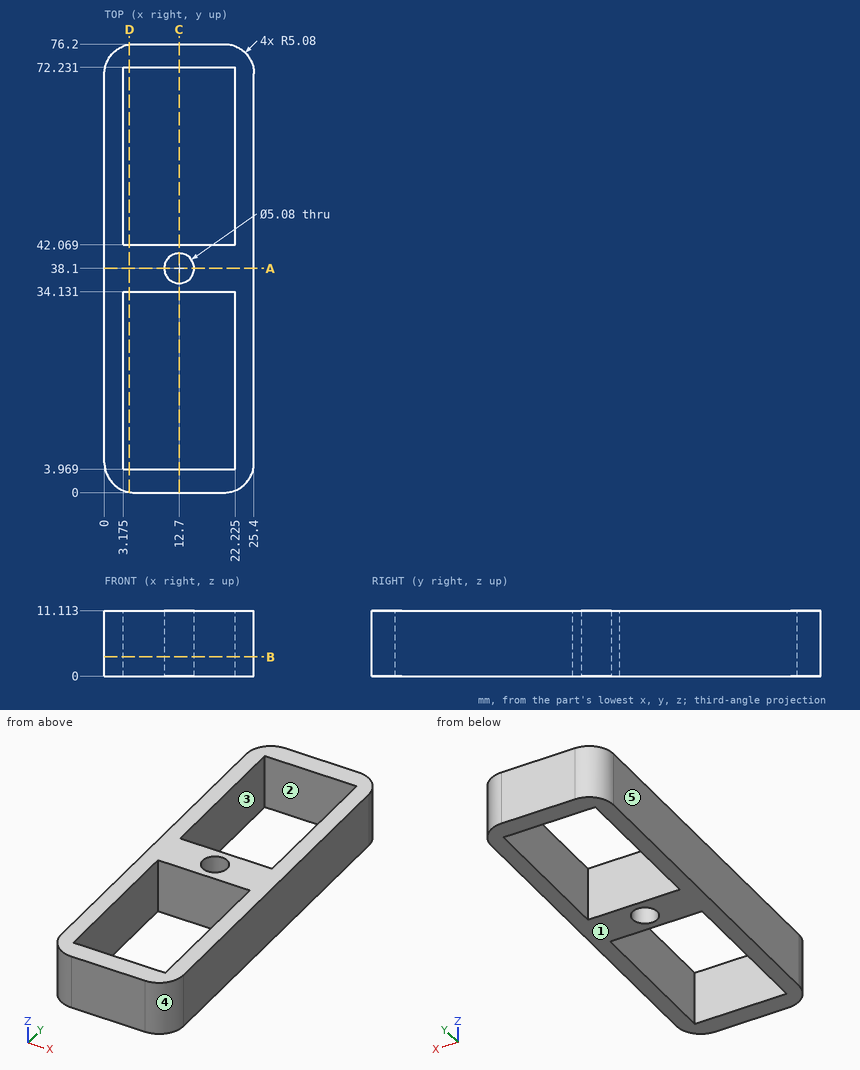
The drawing under review shows one solid part. Ordinate dimensions are in mm from its lowest x, y, z. A direction names the side the tool comes from. Give positions to 0.01 mm unless a question says otherwise; leave off trailing zeros. Loops run counter-clockwise (first coordinate to the right, second up) from the corner with the lowest first, then second, coordinate; pieces in that order, holes last. Notation, with made-up numbers: M -33.75,20 L 23.25,20 A20 ccw 23.25,24 Z; hole C 58.5,40.25 d2. An arc over 180 degrees is marked long. One line per question, with ' | ' between items. Start each with the question number.
1. Add section C-C (x = 12.7). Write out the cut boundary in (y, z), plus the area to 3 significant figures.
2. Insertion check: P1, Ø2, axis at x = 20, z = 4, coming from the -Y side; P2, Ø6, axis at x = 9, y = 68, coming from the +Z side. Each pin has a flat end and moves straight along its axis. Give the tip position at first contact, or say it passes through.
3. For the marked faces 1 and 2, list the 3-axis set-ups (+Z, -Z, +X, -X, +Y, -Y) from which the entire face can be reached by the end or side of a thin tool; tool diameter is ignored.
4. The part is to be moulded in two halves that separate along Y. For the marked faces 3, 4 and 5, say which applies: released by +Y, released by -Y, zero draft, split by the parting line, or undercut.
5. To check wall thickness, follow L1, parallel to Y at x = 6.25, z = 7.25; L2, parallel to Y at x = 12.7, z = 3.75; L3, parallel to X at y = 60.5, z = 1 (1 decimal). State the ranges of each line that lie inside material, in increasing order.
6. Add section B-B (z = 3.25). Write out the cut boundary in (x, y) (1 decimal).
7. Add section A-A (y = 38.1). Write out the cut boundary in (x, z), plus the area to 3 significant figures.
8. Add section D-D (x = 4.25). Write out the cut boundary in (y, z), plus the area to 3 significant figures.
Worked out:
1) outline: M 0,0 L 3.97,0 L 3.97,11.11 L 0,11.11 Z; M 34.13,0 L 35.56,0 L 35.56,11.11 L 34.13,11.11 Z; M 40.64,0 L 42.07,0 L 42.07,11.11 L 40.64,11.11 Z; M 72.23,0 L 76.2,0 L 76.2,11.11 L 72.23,11.11 Z | area: 120 mm²
2) P1: stops at y = 0 | P2: passes through
3) face 1: -Z, +X, -X, +Y, -Y | face 2: +Z, -Z
4) face 3: undercut | face 4: released by -Y | face 5: zero draft
5) L1: y = 0 to 3.97, 34.13 to 42.07, 72.23 to 76.2 | L2: y = 0 to 3.97, 34.13 to 35.56, 40.64 to 42.07, 72.23 to 76.2 | L3: x = 0 to 3.2, 22.2 to 25.4
6) outline: M 0,5.1 A5.1 ccw 5.1,0 L 20.3,0 A5.1 ccw 25.4,5.1 L 25.4,71.1 A5.1 ccw 20.3,76.2 L 5.1,76.2 A5.1 ccw 0,71.1 Z; hole M 3.2,4 L 22.2,4 L 22.2,34.1 L 3.2,34.1 Z; hole M 3.2,42.1 L 22.2,42.1 L 22.2,72.2 L 3.2,72.2 Z; hole C 12.7,38.1 d5.1
7) outline: M 0,0 L 10.16,0 L 10.16,11.11 L 0,11.11 Z; M 15.24,0 L 25.4,0 L 25.4,11.11 L 15.24,11.11 Z | area: 226 mm²
8) outline: M 0.07,0 L 3.97,0 L 3.97,11.11 L 0.07,11.11 Z; M 34.13,0 L 42.07,0 L 42.07,11.11 L 34.13,11.11 Z; M 72.23,0 L 76.13,0 L 76.13,11.11 L 72.23,11.11 Z | area: 175 mm²
